Geometry check sheet. Reference: the model listing, model coordinates, mm. Coordinates: 2 decimals unless noted, no trailing zeros. Write each loop counter-clockwise with the first axis right and the second up, starting at its lowest first coordinate (ties: lowest second). Pieces come first, ordered by that corner, then holes. Notation, with made-up numbers: (38.5, 23) -> (60.5, 23) arc R32 ccw to (60.5, 49) -> close; hole circle Ø8 at (85, 69). An arc over 180 degrees is marked (long way). Answer in a Markdown table with one row per item. Add a question column.
1. Depth check by flat-ended pin: P1, Ø1, axis at y = 160, z = 4.5, coming from the +X side; P2, Ø3, axis at x = 2.5, y = 104, coming from the +Z side; P3, Ø2, axis at x = 13.5, y = 61.5, coming from the +Z side. Enter the tip coordinate at first touch or a pass-through.
2. Cross-section at D-D on z = 3.3. Record the cut outline in (x, y).
3. Cross-section at B-B on x = 13.5. Record the cut outline in (y, z).
4. Scan lines: L1, parallel to Y at x = 2.5, z = 1.55; L2, parallel to X at y = 120.5, z = 1.7; L3, parallel to X at y = 109, z = 3.6. Record each from-to range of solid material in increasing order. Write a range as from..to.
5. Cross-section at C-C on y = 2.5. Record the cut outline in (x, z), and give its area (4 significant figures).
6. Cross-section at A-A on y = 128.5. Record the cut outline in (x, z).
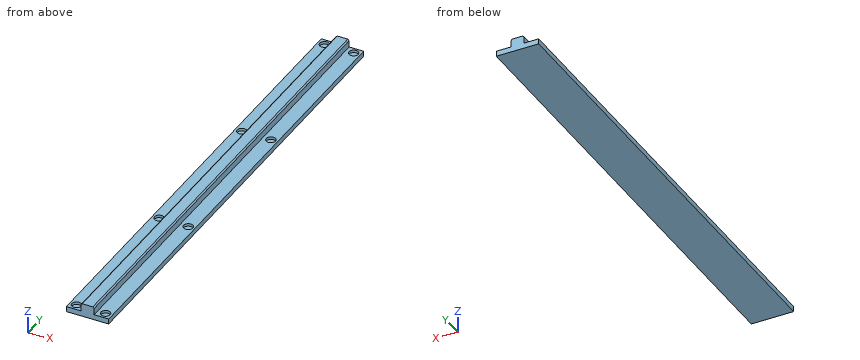
Autodesk Fusion 360 part; units mm, degrees
sketch "3D-printed conduit top outline" plane through (0, 0, 0) normal (0, 1, 0) x (1, 0, 0)
  line L0 (0, 0) -> (16, 0)
  line L1 (16, 0) -> (16, -2)
  line L2 (16, -2) -> (0, -2)
  line L3 (0, -2) -> (0, 0)
  dimension "d7" = 16
  dimension "d8" = 2
extrude "Extrude1" add sketch "3D-printed conduit top outline" along normal blind 182
sketch "Magnet holes" plane through (0, 0, 2) normal (0, 0, 1) x (-1, 0, 0)
  line L0 (0, 0) -> (-16, 0)
  line L1 (-16, 0) -> (-16, -182)
  line L2 (-16, -182) -> (0, -182)
  line L3 (0, -182) -> (0, 0)
  circle A0 centre (-2.5, -2.5) radius 2.5
  circle A1 centre (-13.5, -2.5) radius 2.5
  circle A2 centre (-2.5, -2.5) radius 1.75
  circle A3 centre (-13.5, -2.5) radius 1.75
  circle A4 centre (-2.5, -61.5) radius 1.75
  circle A5 centre (-2.5, -61.5) radius 2.5
  circle A6 centre (-13.5, -61.5) radius 2.5
  circle A7 centre (-13.5, -61.5) radius 1.75
  circle A8 centre (-2.5, -120.5) radius 1.75
  circle A9 centre (-2.5, -120.5) radius 2.5
  circle A10 centre (-13.5, -120.5) radius 2.5
  circle A11 centre (-13.5, -120.5) radius 1.75
  circle A12 centre (-2.5, -179.5) radius 1.75
  circle A13 centre (-2.5, -179.5) radius 2.5
  circle A14 centre (-13.5, -179.5) radius 2.5
  circle A15 centre (-13.5, -179.5) radius 1.75
  dimension "d11" = 5
  dimension "d12" = 5
  dimension "d13" = 3.5
  dimension "d14" = 3.5
  dimension "d17" = 0
  dimension "d18" = -177
extrude "Extrude2" cut sketch "Magnet holes" against normal blind 1 contours A2 | A3 | A4 | A7 | A8 | A11 | A12 | A15
sketch "Support rib" plane through (0, 0, 2) normal (0, 0, 1) x (-1, 0, 0)
  line L0 (0, 0) -> (-16, 0)
  line L1 (-16, 0) -> (-16, -182)
  line L2 (-16, -182) -> (0, -182)
  line L3 (0, -182) -> (0, 0)
  circle A0 centre (-13.5, -179.5) radius 1.75
  circle A1 centre (-13.5, -61.5) radius 1.75
  circle A2 centre (-2.5, -2.5) radius 1.75
  circle A3 centre (-2.5, -120.5) radius 1.75
  circle A4 centre (-2.5, -179.5) radius 1.75
  circle A5 centre (-2.5, -61.5) radius 1.75
  circle A6 centre (-13.5, -2.5) radius 1.75
  circle A7 centre (-13.5, -120.5) radius 1.75
  line L4 (-5.5, 0) -> (-10.5, 0)
  line L5 (-10.5, 0) -> (-10.5, -182)
  line L6 (-10.5, -182) -> (-5.5, -182)
  line L7 (-5.5, -182) -> (-5.5, 0)
  dimension "d23" = 5
  dimension "d24" = 5.5
  dimension "d25" = 5.5
extrude "Extrude3" add sketch "Support rib" along normal blind 3 contours L0 L2 L4 L5 L6 L7
chamfer "Chamfer1" distance 0.5 angle 45 2 edges at (5.5, 91, 5) (10.5, 91, 5)
equation "conduit_length = 182.00 mm"
equation "conduit_width = 16 mm"
equation "conduit_wall_thickness = 2 mm"
equation "magnet_diameter = 3 mm"
equation "magnet_height = 1 mm"
equation "d7 = conduit_width"
equation "d8 = conduit_wall_thickness"
equation "d9 = conduit_length"
equation "d11 = magnet_diameter + 2 mm"
equation "d12 = magnet_diameter + 2 mm"
equation "d13 = magnet_diameter + 0.5 mm"
equation "d14 = magnet_diameter + 0.5 mm"
equation "d18 = -conduit_length + magnet_diameter + 2 mm"
equation "rib_width = 5 mm"
equation "rib_height = 3 mm"
equation "d23 = rib_width"
equation "d24 = ( conduit_width - rib_width ) / 2"
equation "d26 = rib_height"
equation "rib_chamfer = 0.5 mm"
equation "d29 = rib_chamfer"
Results found:
| question | item | result |
|---|---|---|
| 1 | P1 | stops at x = 10.5 |
| 1 | P2 | stops at z = 2 |
| 1 | P3 | stops at z = 1 |
| 2 | outline | (5.5, 0) -> (10.5, 0) -> (10.5, 182) -> (5.5, 182) -> close |
| 3 | outline | (0, 0) -> (182, 0) -> (182, 2) -> (181.25, 2) -> (181.25, 1) -> (177.75, 1) -> (177.75, 2) -> (122.25, 2) -> (122.25, 1) -> (118.75, 1) -> (118.75, 2) -> (63.25, 2) -> (63.25, 1) -> (59.75, 1) -> (59.75, 2) -> (4.25, 2) -> (4.25, 1) -> (0.75, 1) -> (0.75, 2) -> (0, 2) -> close |
| 4 | L1 | y = 0..0.75, 4.25..59.75, 63.25..118.75, 122.25..177.75, 181.25..182 |
| 4 | L2 | x = 0..0.75, 4.25..11.75, 15.25..16 |
| 4 | L3 | x = 5.5..10.5 |
| 5 | outline | (0, 0) -> (16, 0) -> (16, 2) -> (15.25, 2) -> (15.25, 1) -> (11.75, 1) -> (11.75, 2) -> (10.5, 2) -> (10.5, 4.5) -> (10, 5) -> (6, 5) -> (5.5, 4.5) -> (5.5, 2) -> (4.25, 2) -> (4.25, 1) -> (0.75, 1) -> (0.75, 2) -> (0, 2) -> close |
| 5 | area | 39.75 mm^2 |
| 6 | outline | (0, 0) -> (16, 0) -> (16, 2) -> (10.5, 2) -> (10.5, 4.5) -> (10, 5) -> (6, 5) -> (5.5, 4.5) -> (5.5, 2) -> (0, 2) -> close |
